Can you work these out from the model? Positions are in its coordinate system, mm. Face numbers are marked on the shaded views. A direction names the side the tool comes from. Round coordinates to 2 decimals unless told otherwise and drop trailing zeros. Order: outer loops, then holes, each group sorted by start corner. A loop starts at its lowest first (then second) coordinate and runs counter-clockwise, first axis right, second up.
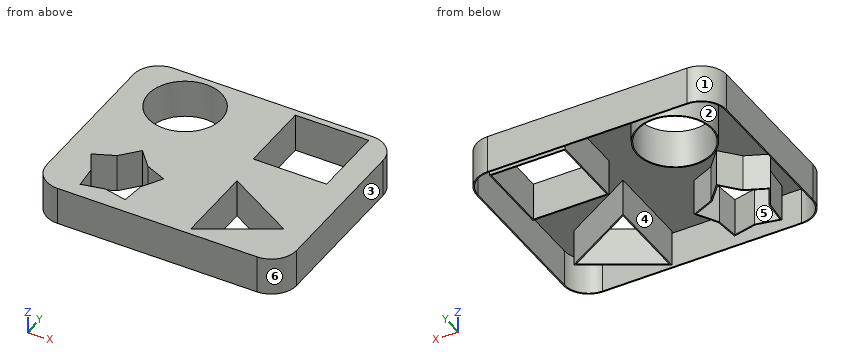
Autodesk Inventor part; units mm, degrees
ref_plane "YZ Plane" through (0, 0, 0) normal (1, 0, 0) x (0, 1, 0)
ref_plane "XZ Plane" through (0, 0, 0) normal (0, 1, 0) x (-1, 0, 0)
ref_plane "XY Plane" through (0, 0, 0) normal (0, 0, 1) x (1, 0, 0)
sketch "Sketch1" plane through (0, 0, 0) normal (0, 0, 1) x (1, 0, 0)
  line L0 (0, 0) -> (50.165, 0)
  line L1 (50.165, 0) -> (50.165, 40.386)
  line L2 (50.165, 40.386) -> (0, 40.386)
  line L3 (0, 40.386) -> (0, 0)
  dimension "d0" = 50.165
  dimension "d1" = 40.386
extrude "Extrusion1" add sketch "Sketch1" along normal blind 7.62
sketch "Sketch2" plane through (0, 0, 7.62) normal (0, 0, 1) x (1, 0, 0)
  circle A0 centre (12.446, 31.75) radius 7.366
  line L0 (0, 40.386) -> (0, 0)
  line L1 (50.165, 40.386) -> (0, 40.386)
  line L2 (30.353, 39.116) -> (45.085, 39.116)
  line L3 (45.085, 39.116) -> (45.085, 24.384)
  line L4 (45.085, 24.384) -> (30.353, 24.384)
  line L5 (30.353, 24.384) -> (30.353, 39.116)
  line L6 (50.165, 0) -> (50.165, 40.386)
  line L7 (31.0509, 1.27) -> (31.0509, 17.4752)
  line L8 (31.0509, 17.4752) -> (45.085, 9.3726)
  line L9 (45.085, 9.3726) -> (31.0509, 1.27)
  line L10 (0, 0) -> (50.165, 0)
  circle A1 centre (12.3952, 9.2202) radius 7.6835 construction
  line L11 (12.3952, 16.9037) -> (19.7026, 11.5945) construction
  line L12 (19.7026, 11.5945) -> (16.9114, 3.0041) construction
  line L13 (16.9114, 3.0041) -> (7.879, 3.0041) construction
  line L14 (7.879, 3.0041) -> (5.0878, 11.5945) construction
  line L15 (5.0878, 11.5945) -> (12.3952, 16.9037) construction
  circle A2 centre (12.3952, 9.2202) radius 5.2324 construction
  line L16 (12.3952, 16.9037) -> (9.3197, 13.4533)
  line L17 (9.3197, 13.4533) -> (5.0878, 11.5945)
  line L18 (5.0878, 11.5945) -> (7.4189, 7.6033)
  line L19 (7.4189, 7.6033) -> (7.879, 3.0041)
  line L20 (7.879, 3.0041) -> (12.3952, 3.9878)
  line L21 (16.9114, 3.0041) -> (12.3952, 3.9878)
  line L22 (16.9114, 3.0041) -> (17.3715, 7.6033)
  line L23 (17.3715, 7.6033) -> (19.7026, 11.5945)
  line L24 (12.3952, 16.9037) -> (15.4707, 13.4533)
  line L25 (19.7026, 11.5945) -> (15.4707, 13.4533)
  point P0 (35.7289, 9.3726)
  dimension "d4" = 14.732
  dimension "d5" = 12.446
  dimension "d6" = 8.636
  dimension "d7" = 14.732
  dimension "d8" = 5.08
  dimension "d9" = 1.27
  dimension "d10" = 14.732
  dimension "d11" = 16.2052
  dimension "d12" = 1.27
  dimension "d13" = 5.08
  dimension "d14" = 15.367
  dimension "d15" = 12.3952
  dimension "d16" = 9.2202
  dimension "d17" = 10.4648
extrude "Extrusion2" cut sketch "Sketch2" against normal blind 25.4 contours A0 | L2 L3 L4 L5 | L7 L8 L9 | L24 L25 L23 L22 L21 L20 L19 L18 L17 L16
fillet "Fillet1" radius 5.08 1 edges at (50.165, 40.386, 3.81)
fillet "Fillet2" radius 5.08 1 edges at (0, 40.386, 3.81)
fillet "Fillet3" radius 5.08 1 edges at (50.165, 0, 3.81)
fillet "Fillet4" radius 5.08 1 edges at (0, 0, 3.81)
shell "Shell1" thickness 0.254 removed faces 1 at (40.407, 17.0773, 0)
properties part number "PassengerBaseNT"
(1) If we mould it in two halves opening along Y, with no side actions, what happens to the marked faces 1, 2 and 3? For each: pulls with the +Y half, pulls with the -Y half, needs draft (parallel to the pull), parting line crosses it, or undercut.
(2) On a 3-axis mill with a long thin cutter (end or side, diameter ignored), from which of +Z, -Z, +X, -X, +Y, -Y can I reach the whole of each face in a straight line? I mean the marked faces 4, 5 and 6. Say none if no direction works.
(3) Please list where these lines run through material, in increasing order: probe 1 along X at (y, z) = (22, 7) (3 decimals); probe 2 along Y at (x, z) = (24, 1); probe 3 along X at (y, z) = (36, 2) (3 decimals).
(4) I want a section at B-B, the plane x = 18.5. List the corners of the cut face in (y, z) for me.
(5) I want a section at D-D, the plane y = 22. List the corners of the cut face in (x, z) for me (3 decimals).
(6) I want a section at C-C, the plane z = 5.5. Give the number of separate pieces and of enclosed holes in the cut face, plus the area to 3 significant figures.
(7) I want a section at A-A, the plane y = 31.75. List the corners of the cut face in (x, z) for me (3 decimals).
Ans:
1. face 1: pulls with the +Y half
1. face 2: undercut
1. face 3: needs draft
2. face 4: -Z
2. face 5: +Z, -Z
2. face 6: +Z, -Z, +X, -Y
3. probe 1: x = 0 to 0.254, 49.911 to 50.165
3. probe 2: y = 0 to 0.25, 40.13 to 40.39
3. probe 3: x = 0.048 to 0.304, 6.121 to 6.43, 18.462 to 18.771, 30.099 to 30.353, 45.085 to 45.339, 49.861 to 50.117
4. outline: (0, 0) - (0.25, 0) - (0.25, 7.37) - (9.03, 7.37) - (9.03, 0) - (9.54, 0) - (9.54, 7.62) - (0, 7.62) - close; (12.12, 0) - (12.4, 0) - (12.4, 7.37) - (27.12, 7.37) - (27.12, 0) - (27.55, 0) - (27.55, 7.62) - (12.12, 7.62) - close; (35.95, 0) - (36.38, 0) - (36.38, 7.37) - (40.13, 7.37) - (40.13, 0) - (40.39, 0) - (40.39, 7.62) - (35.95, 7.62) - close
5. outline: (0, 0) - (0.254, 0) - (0.254, 7.366) - (49.911, 7.366) - (49.911, 0) - (50.165, 0) - (50.165, 7.62) - (0, 7.62) - close
6. separate pieces: 5
6. enclosed holes: 5
6. area: 95.5 mm2
7. outline: (0, 0) - (0.254, 0) - (0.254, 7.366) - (4.826, 7.366) - (4.826, 0) - (5.08, 0) - (5.08, 7.62) - (0, 7.62) - close; (19.812, 0) - (20.066, 0) - (20.066, 7.366) - (30.099, 7.366) - (30.099, 0) - (30.353, 0) - (30.353, 7.62) - (19.812, 7.62) - close; (45.085, 0) - (45.339, 0) - (45.339, 7.366) - (49.911, 7.366) - (49.911, 0) - (50.165, 0) - (50.165, 7.62) - (45.085, 7.62) - close
